from build123d import *

# Parameters (mm, degrees)
SKETCH1_R           = 20
BOSS_EXTRUDE1_DEPTH = 5
SKETCH2_R           = 2
CUT_EXTRUDE1_DEPTH  = 30
SKETCH3_R           = 4
BOSS_EXTRUDE3_DEPTH = 40
SKETCH4_R           = 2.5
CUT_EXTRUDE2_DEPTH  = 16


with BuildPart() as part:
    # Sketch1 → Boss-Extrude1 (new body)
    with BuildSketch(Plane.XY):
        with Locations((-0.483808042, 0)):
            Circle(SKETCH1_R)
    extrude(amount=BOSS_EXTRUDE1_DEPTH)

    # Sketch2 → Cut-Extrude1 (cut)
    with BuildSketch(Plane(origin=(0, 0, 0), x_dir=(-1, 0, 0), z_dir=(0, 0, -1))):
        with Locations((7.5, 7.5)):
            Circle(SKETCH2_R)
        with Locations((7.5, -7.5)):
            Circle(SKETCH2_R)
        with Locations((-7.5, -7.5)):
            Circle(SKETCH2_R)
        with Locations((-7.5, 7.5)):
            Circle(SKETCH2_R)
    extrude(amount=-CUT_EXTRUDE1_DEPTH, mode=Mode.SUBTRACT)

    # Sketch3 → Boss-Extrude3 (add)
    with BuildSketch(Plane(origin=(0, 0, 0), x_dir=(-1, 0, 0), z_dir=(0, 0, -1))):
        Circle(SKETCH3_R)
    extrude(amount=BOSS_EXTRUDE3_DEPTH)

    # Sketch4 → Cut-Extrude2 (cut)
    with BuildSketch(Plane(origin=(0, 0, -40), x_dir=(-1, 0, 0), z_dir=(0, 0, -1))):
        Circle(SKETCH4_R)
    extrude(amount=-CUT_EXTRUDE2_DEPTH, mode=Mode.SUBTRACT)


solid = part.part
Could you check a few things on this model? Use its own coordinates, in mm. A direction names the side the tool comes from. Round coordinates to 2 decimals unless told otherwise and drop trailing zeros. Order: outer loops, then holes, each group sorted by start corner. A loop starts at its lowest first (then second) coordinate and runs counter-clockwise, first axis right, second up. Notation, with made-up numbers: M 53.5,47 L 72.5,47 A21 cw 72.5,81 Z; hole C -4.5,27 d6. An arc over 180 degrees is marked long. One line per item, written item: value.
(1) I need wall thicknesses on line 1 along Y through (x, z) = (0, -36); line 2 along Y through (x, z) = (-7, 3); line 3 along Y through (x, z) = (7.5, 1.25). Which ranges of each line are inside material? Lowest first, please. Write a range as from..to.
Ans:
line 1: y = -4..-2.5, 2.5..4
line 2: y = -18.91..-9.44, -5.56..5.56, 9.44..18.91
line 3: y = -18.34..-9.5, -5.5..5.5, 9.5..18.34
(2) Which directions (+Z, -Z, +X, -X, +Y, -Y) give clear straight access to the entire face, cutting with the end or side of a thin tool? Please do faces 1 (the cylindrical face through (0.54, -2.44, -32.11)), 2 (the cylindrical face through (8.974, 8.852, 2.465)).
Ans:
face 1: -Z
face 2: +Z, -Z
(3) Imagine slicing it at B-B (x = 7.5). Write out the boundary of the cut face in (y, z).
Ans:
outline: M -18.34,0 L -9.5,0 L -9.5,5 L -18.34,5 Z; M -5.5,0 L 5.5,0 L 5.5,5 L -5.5,5 Z; M 9.5,0 L 18.34,0 L 18.34,5 L 9.5,5 Z
(4) I'm going to push flat-ended pins straight in: P1, Ø2.5, axis at x = -7.5, y = -7.5, coming from the -Z side; P2, Ø4, axis at y = 1, z = -15.5, coming from the +X side; P3, Ø4, axis at x = 4.5, z = -25, coming from the +Y side; P4, Ø5, axis at x = -12.5, y = 13.5, coming from the -Z side. Where does each tip first touch, or does it pass through?
Ans:
P1: passes through
P2: stops at x = 4
P3: stops at y = 3.12
P4: stops at z = 0
(5) Imagine slicing it at A-A (y = 0). Write out the boundary of the cut face in (x, z).
Ans:
outline: M -20.48,0 L -4,0 L -4,-40 L -2.5,-40 L -2.5,-24 L 2.5,-24 L 2.5,-40 L 4,-40 L 4,0 L 19.52,0 L 19.52,5 L -20.48,5 Z
(6) If we mould it in two halves opening along Y, with no side actions, what happens to faces 3 (the flat face through (-1, 0, 5)), 4 (the cylindrical face through (-4.819, -19.524, 2.465)), 5 (the cylindrical face through (-6.026, 8.852, 2.465))? For each: released by +Y, released by -Y, zero draft, split by the parting line, or undercut.
Ans:
face 3: zero draft
face 4: split by the parting line
face 5: undercut
(7) Imagine slicing it at C-C (y = -7.5). Write out the boundary of the cut face in (x, z).
Ans:
outline: M -19.02,0 L -9.5,0 L -9.5,5 L -19.02,5 Z; M -5.5,0 L 5.5,0 L 5.5,5 L -5.5,5 Z; M 9.5,0 L 18.06,0 L 18.06,5 L 9.5,5 Z
(8) Imagine slicing it at D-D (z = -36.5). Write out the boundary of the cut face in (x, y), and give its area (3 significant figures).
Ans:
outline: C 0,0 d8; hole C 0,0 d5
area: 30.6 mm^2
